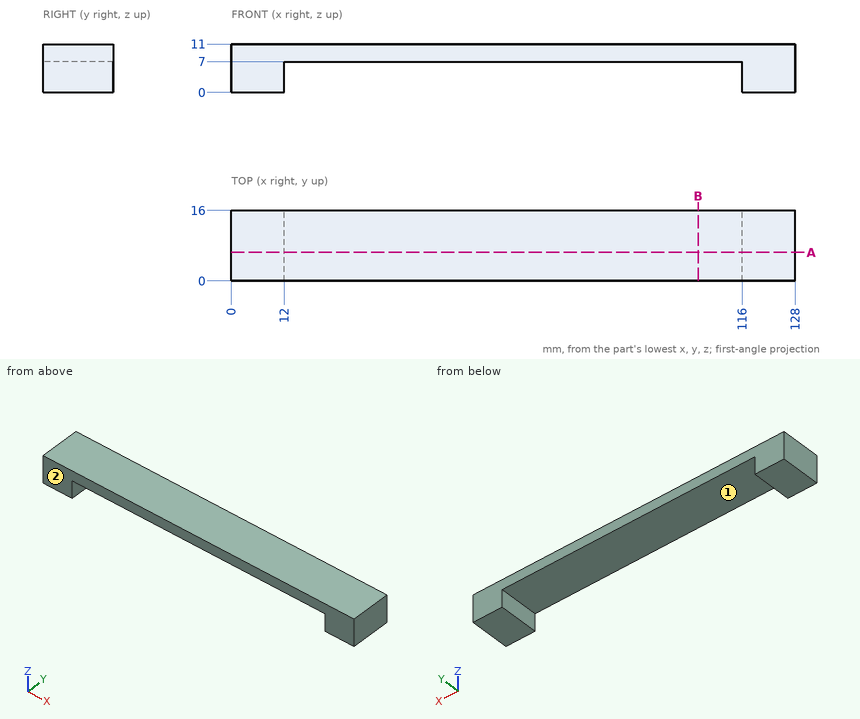
Job drawing, mm, ordinate dimensions from the low corner. One solid piece. A direction names the side the tool comes from. Coordinates: 2 decimals unless noted, no trailing zeros. Write each loop counter-clockwise with the first axis right and the second up, starting at its lowest first coordinate (ties: lowest second). Pieces come first, ordered by that corner, then holes. Notation, with made-up numbers: (82, 55) -> (137, 55) arc R18 cw to (137, 84) -> close; hole circle Ø5 at (-32, -37.75). An arc over 180 degrees is marked (long way). Use CSV: the item, a comma, the result in double quotes. Start each with the question number.
Item 1: Band-saw the part on A-A, the plane y = 6.5. Write the cut outline in (x, z), plus the area to 3 significant figures.
Item 2: Tool access for the marked faces 1 and 2: list every direction of +Z, -Z, +X, -X, +Y, -Y with a clear straight run to the whole face (end or side of a thin tool).
Item 3: Band-saw the part on B-B, the plane x = 106. Write the cut outline in (y, z).
Item 4: Wall check: probe 1 along X at (y, z) = (5.5, 1.5); probe 2 along Z at (x, y) = (80.5, 6.25). Give the ranges that are in metal, low to high.
Item 5: Drop a flat-ended pin along its axis: P1, Ø6, axis at x = 33, y = 13.5, coming from the -Z side. Give the stop position or say it passes through.
Response values:
1,outline,"(0, 0) -> (12, 0) -> (12, 7) -> (116, 7) -> (116, 0) -> (128, 0) -> (128, 11) -> (0, 11) -> close"
1,area,"680 mm2"
2,face 1,"-Z, +Y, -Y"
2,face 2,"+Z, -Z, +X, -X, -Y"
3,outline,"(0, 7) -> (16, 7) -> (16, 11) -> (0, 11) -> close"
4,probe 1,"x = 0 to 12, 116 to 128"
4,probe 2,"z = 7 to 11"
5,P1,"stops at z = 7"
